Input: part model. Units: mm. Frame: model coordinates. Coordinates: 2 decimals unless noted, no trailing zeros. Order: outer loops, then holes, each group sorted by start corner. A loop starts at its lowest first (then second) coordinate and runs counter-clockwise, first axis right, second up. Notation, with made-up numbers: (-17.5, 65) - (27.5, 65) arc R31 cw to (27.5, 99) - close; hole circle Ø9 at (32.5, 73). An arc over 180 degrees is marked (long way). Answer as CSV lines item,"result". Start each with the question number.
Item 1: Section C-C (y = -39.5). Output: boundary loops of the cut face in (x, z).
Item 2: Section D-D (z = 36). Output: boundary loops of the cut face in (x, y), and give its area (3 significant figures).
Item 3: First-contact query: pin 1 (4 mm diameter, centred on x = -19, y = 19, fed in from -Z); pin 2 (1.5 mm diameter, centred on x = -2, y = -26, fed in from +Z); pin 3 (10 mm diameter, centred on x = 0, y = 0, fed in from +Z); pin 4 (10 mm diameter, centred on y = -3, z = 59.5, fed in from +X). Flat tips, straight axial feed; report the tip coordinate or a pass-through.
Item 4: Section A-A (y = 0). Output: boundary loops of the cut face in (x, z), and give its area (3 significant figures).
Item 5: Section B-B (x = 0). Output: boundary loops of the cut face in (y, z).
Item 6: Draft query along Y for faces 1 (the flat face through (83.01, -10.93, 35.23)), 2 (the cylindrical face through (-1.38, -6.2, 2.46)), 3 (the flat face through (-1, -10, 5)), 4 (the conical face through (85, 0, 40)). Return one class per face: +Y half, -Y half, draft (parallel to the pull), parting line (faces both ways), or undercut.
Item 7: Material intervals for line 1 along Y through (x, z) = (0, 2.8); line 2 along Z through (x, y) = (33, -35.5); line 3 along X through (y, z) = (0.5, 50), sorted ascending.
from build123d import *

# Parameters (mm, degrees)
F0_R     = 50
F0_R_2   = 6.35
F1_DEPTH = 5
F3_ANGLE = 15


with BuildPart() as f1:
    # F0 (on Top) → F1 (new body)
    with BuildSketch(Plane.XY):
        Circle(F0_R)
        Circle(F0_R_2, mode=Mode.SUBTRACT)
    extrude(amount=F1_DEPTH)

    # F2 (on Front) → F3 (revolve, symmetric)
    with BuildSketch(Plane.XZ) as f3_sk:
        Polygon((120.710678, 75.710678), (50, 5), (50, 0), (123.210678, 73.210678), align=None)
    revolve(axis=Axis((0, 0, 11.425557), (0, 0, 1)), revolution_arc=F3_ANGLE / 2)
    revolve(f3_sk.sketch, axis=Axis((0, 0, 11.425557), (0, 0, -1)), revolution_arc=F3_ANGLE / 2)


solid = f1.part
Determined:
1,outline,"(-30.66, 0) - (30.66, 0) - (30.66, 5) - (-30.66, 5) - close"
2,outline,"(80.31, -10.57) - (85.26, -11.23) arc R86 ccw to (85.26, 11.23) - (80.31, 10.57) arc R81 cw to start"
2,area,"109 mm^2"
3,pin 1,"stops at z = 0"
3,pin 2,"stops at z = 5"
3,pin 3,"passes through"
3,pin 4,"stops at x = 114.46"
4,outline,"(-50, 0) - (-6.35, 0) - (-6.35, 5) - (-50, 5) - close; (6.35, 0) - (50, 0) - (123.21, 73.21) - (120.71, 75.71) - (50, 5) - (6.35, 5) - close"
4,area,"796 mm^2"
5,outline,"(-50, 0) - (-6.35, 0) - (-6.35, 5) - (-50, 5) - close; (6.35, 0) - (50, 0) - (50, 5) - (6.35, 5) - close"
6,face 1,"-Y half"
6,face 2,"undercut"
6,face 3,"draft"
6,face 4,"undercut"
7,line 1,"y = -50 to -6.35, 6.35 to 50"
7,line 2,"z = 0 to 5"
7,line 3,"x = 95 to 100"
